Autodesk Inventor part; units mm, degrees
ref_plane "YZ Plane" through (0, 0, 0) normal (1, 0, 0) x (0, 1, 0)
ref_plane "XZ Plane" through (0, 0, 0) normal (0, 1, 0) x (-1, 0, 0)
ref_plane "XY Plane" through (0, 0, 0) normal (0, 0, 1) x (1, 0, 0)
sketch "草图1" plane through (0, 0, 0) normal (0, 0, 1) x (1, 0, 0)
  line L0 (80.5, -10) -> (-80.5, -10)
  line L1 (-80.5, -10) -> (-80.5, 10)
  line L2 (-80.5, 10) -> (80.5, 10)
  line L3 (80.5, 10) -> (80.5, -10)
  line L4 (80.5, -10) -> (-80.5, 10) construction
  line L5 (-80.5, -10) -> (80.5, 10) construction
  point P0 (0, 0)
  dimension "d0" = 20
  dimension "d1" = 161
extrude "拉伸1" add sketch "草图1" along normal blind 3
sketch "草图2" plane through (0, 0, 3) normal (0, 0, 1) x (1, 0, 0)
  circle A0 centre (73.5, 2.1994) radius 1.5
  line L0 (80.5, 10) -> (-80.5, 10)
  line L1 (80.5, -10) -> (80.5, 10)
  line L2 (-80.5, 10) -> (80.5, 10)
  line L3 (0, 10) -> (0, -10)
  line L4 (-80.5, -10) -> (80.5, -10)
  circle A1 centre (-73.5, 2.1994) radius 1.5
  point P0 (0, 0)
extrude "拉伸2" cut sketch "草图2" against normal blind 10 contours A0 | A1
properties part number "前挡板"
Source: CAD feature listing. Evaluate the final solid. Frame: model axes, mm. Coordinates: 2 decimals unless noted, no trailing zeros. Write each loop counter-clockwise with the first axis right and the second up, starting at its lowest first coordinate (ties: lowest second). Pieces come first, ordered by that corner, then holes. Notation, with made-up numbers: M 58,-25 L 83,-25 A18 ccw 83,1 Z; hole C 26.5,-26 d1. An arc over 180 degrees is marked long. Answer as a JSON object with one key per item and string values.
1. Draft query along X for faces 1 (the flat face through (-1, 0, 0)), 2 (the flat face through (80.5, 0, 1)), 3 (the cylindrical face through (74.93, 2.65, 1.52)). Return one class per face: released by +X, released by -X, zero draft, split by the parting line, or undercut.
Evaluation:
{"face 1": "zero draft", "face 2": "released by +X", "face 3": "undercut"}
2. Ray query, L1, parallel to Y at x = -73.5, z = 2.15. Return the intervals inside material, ascending.
Evaluation:
{"L1": "-10 to 0.7, 3.7 to 10"}
3. Cut plane A-A on x = -73.5. Output: boundary loops of the cut face in (y, z), plus the area to 3 significant figures.
Evaluation:
{"outline": "M -10,0 L 0.7,0 L 0.7,3 L -10,3 Z; M 3.7,0 L 10,0 L 10,3 L 3.7,3 Z", "area": "51.0 mm^2"}
